from build123d import *

# Parameters (mm, degrees)
F0_W     = 450
F0_H     = 450
F1_DEPTH = 950
F2_W     = 50
F2_H     = 315.0687813759
F2_W_2   = 326.7514157295
F3_DEPTH = 450.001
F5_DEPTH = 400.001
F6_W     = 380
F6_H     = 412.3499316829
F6_H_2   = 50
F7_DEPTH = 120.98296301


with BuildPart() as f1:
    # F0 (on Top) → F1 (new body)
    with BuildSketch(Plane.XY):
        Rectangle(F0_W, F0_H)
    extrude(amount=F1_DEPTH)

    # F2 (on face) → F3 (cut, through all)
    with BuildSketch(Plane.XZ.offset(225)):
        Polygon((-225, 950), (-225, 365.0687813759), (136.7514157295, 365.0687813759), (190, 950), align=None)
        Polygon((200, 657.5343906879), (175, 365.0687813759), (225, 365.0687813759), (225, 950), align=None)
        Polygon((225, 365.0687813759), (175, 365.0687813759), (175, 315.0687813759), (225, 315.0687813759), (225, 360.064893961), (225, 365.064893961), align=None)
        with Locations((200, 157.5343906879)):
            Rectangle(F2_W, F2_H)
        with Locations((-26.6242921352, 157.5343906879)):
            Rectangle(F2_W_2, F2_H)
    extrude(amount=-F3_DEPTH, mode=Mode.SUBTRACT)

    # F4 (on face) → F5 (cut, through all)
    with BuildSketch(Plane.YZ.offset(175)):
        Polygon((-190, 172.1675388782), (-190, 0), (190, 0), (190, 330.3755388782), (-190, 330.3755388782), align=None)
    extrude(amount=-F5_DEPTH, mode=Mode.SUBTRACT)

    # F6 (on face) → F7 (cut, through all)
    with BuildSketch(Plane(origin=(102.6669528821, 0, -9.3461756156), x_dir=(0, -1, 0), z_dir=(-0.9958819897, 0, 0.0906590457))):
        with Locations((0, 582.1381430631)):
            Rectangle(F6_W, F6_H)
        with Locations((0, 863.3131089045)):
            Rectangle(F6_W, F6_H_2)
    extrude(amount=-F7_DEPTH, mode=Mode.SUBTRACT)


solid = f1.part
Source: CAD feature listing. Evaluate the final solid. Frame: model axes, mm. A direction names the side the tool comes from. Give positions to 0.01 mm unless a question says otherwise; leave off trailing zeros. Write each loop counter-clockwise with the first axis right and the second up, starting at its lowest first coordinate (ties: lowest second). Pieces come first, ordered by that corner, then holes. Notation, with made-up numbers: M 62.5,53.25 L 116.5,53.25 A27 ccw 116.5,92.25 Z; hole C 33,56 d8. An arc over 180 degrees is marked long. Answer as a JSON object with one key per item and string values.
Q1. Cut plane B-B, the plane z = 303. Return the cut outline in (x, y).
Geometry check:
{"outline": "M -225,-225 L -190,-225 L -190,-190 L -225,-190 Z; M -225,190 L -190,190 L -190,225 L -225,225 Z; M 136.75,-225 L 175,-225 L 175,-190 L 136.75,-190 Z; M 136.75,190 L 175,190 L 175,225 L 136.75,225 Z"}
Q2. Ray query, line 1 along Y through (x, z) = (171, 694); line 2 along Z through (x, y) = (-2, -8); line 3 along Z through (x, y) = (-55.5, 203). Return the intervals inside material, ascending.
Geometry check:
{"line 1": "y = -225 to -190, 190 to 225", "line 2": "z = 330.38 to 365.07", "line 3": "z = 315.07 to 365.07"}
Q3. Contact query for a flat-ended pin moving along its axis: P1, Ø6, axis at x = 160.5, y = 84.5, coming from the +Z side. Output: stop coordinate, or through.
Geometry check:
{"P1": "stops at z = 363.18"}
Q4. Cut plane C-C, the plane z = 724. Return the cut outline in (x, y).
Geometry check:
{"outline": "M 169.43,-225 L 205.68,-225 L 205.68,-190 L 169.43,-190 Z; M 169.43,190 L 205.68,190 L 205.68,225 L 169.43,225 Z"}
Q5. Cut plane A-A, the plane y = 136. Return the cut outline in (x, z), then the cut area to 3 significant figures.
Geometry check:
{"outline": "M -225,330.38 L 175,330.38 L 175,361.59 L 136.75,365.07 L -225,365.07 Z; M 174.13,775.72 L 209.82,772.47 L 214.08,822.29 L 178.67,825.51 Z; M 183.2,875.31 L 218.34,872.11 L 225,950 L 190,950 Z", "area": "18,300 mm^2"}
Q6. Access query for faces 4 (the face through (-47, -3, 365.069)), 5 (the face through (-225, -1, 344)), 6 (the face through (-190, -208, 155)), 7 (the face through (139, 190, 189)). Directions: +Z, -Z, +X, -X, +Y, -Y. A direction counts if a zero-diameter tool reaches every point of the face in a straight line with its end or side. Return the directions, or none.
Geometry check:
{"face 4": "+Z, -X, +Y, -Y", "face 5": "+Z, -Z, -X, +Y, -Y", "face 6": "-Z, +Y, -Y", "face 7": "-Z, +X, -X"}
Q7. Cut plane D-D, the plane x = -5.5. Return the cut outline in (y, z).
Geometry check:
{"outline": "M -225,315.07 L -190,315.07 L -190,330.38 L 190,330.38 L 190,315.07 L 225,315.07 L 225,365.07 L -225,365.07 Z"}
Q8. Mould query, pull axis Z, two halves, no side actions, for faces 1 (the face through (207, 3, 950)), 2 (the face through (136.751, 207, 155)), 3 (the face through (198, 190, 848)). Classes: +Z half, -Z half, draft (parallel to the pull), parting line (faces both ways), or undercut.
Geometry check:
{"face 1": "+Z half", "face 2": "draft", "face 3": "undercut"}
